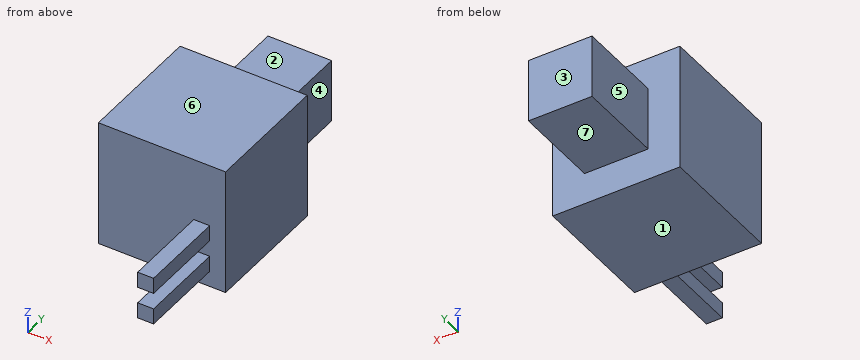
```python
from build123d import *

# Parameters (mm, degrees)
SKETCH1_W           = 8
SKETCH1_H           = 8
BOSS_EXTRUDE1_DEPTH = 8
SKETCH2_W           = 4
SKETCH2_H           = 4
BOSS_EXTRUDE2_DEPTH = 5.5
SKETCH3_W           = 1
SKETCH3_H           = 1
BOSS_EXTRUDE3_DEPTH = 5.5


with BuildPart() as part:
    # Sketch1 → Boss-Extrude1 (new body)
    with BuildSketch(Plane(origin=(0, 0, 0), x_dir=(1, 0, 0), z_dir=(0, 1, 0))):
        Rectangle(SKETCH1_W, SKETCH1_H)
    extrude(amount=BOSS_EXTRUDE1_DEPTH)

    # Sketch2 → Boss-Extrude2 (add)
    with BuildSketch(Plane(origin=(0, 8, 0), x_dir=(1, 0, 0), z_dir=(0, 1, 0))):
        Rectangle(SKETCH2_W, SKETCH2_H)
    extrude(amount=BOSS_EXTRUDE2_DEPTH)

    # Sketch3 → Boss-Extrude3 (add)
    with BuildSketch(Plane.XZ):
        with Locations((2.5, -2.5)):
            Rectangle(SKETCH3_W, SKETCH3_H)
        with Locations((2.5, -0.47334968)):
            Rectangle(SKETCH3_W, SKETCH3_H)
    extrude(amount=BOSS_EXTRUDE3_DEPTH)


solid = part.part
```
Could you check a few things on this model? Use its own coordinates, in mm. Face numbers are marked on the shaded views. A direction names the side the tool comes from. Coordinates: 2 decimals unless noted, no trailing zeros. Write each loop counter-clockwise with the first axis right and the second up, starting at its lowest first coordinate (ties: lowest second). Pieces come first, ordered by that corner, then holes. Notation, with made-up numbers: (40.5, 12) -> (92.5, 12) arc R32 ccw to (92.5, 46) -> close; hole circle Ø10 at (38.5, -14.75). An arc over 180 degrees is marked (long way). Write item = value, one per line. Start each with the question number.
(1) I want a section at B-B (z = -1.75). Please give me the cut outline in (x, y), plus the area to 3 significant figures.
(2) I want a section at A-A (x = 0). Please give me the cut outline in (y, z), plus the area to 3 significant figures.
(3) Which directions (+Z, -Z, +X, -X, +Y, -Y) give clear straight access to the entire face, cutting with the end or side of a thin tool? Please do the marked faces 4, 5, 6 and 7.
(4) I want a section at D-D (z = -0.25). Please give me the cut outline in (x, y), plus the area to 3 significant figures.
(5) I need wall thicknesses on line 1 (X direction, y = 10, z = 1); line 2 (Y direction, x = 2.5, z = -2.5); line 3 (Y direction, x = 0.75, z = 1). Which ranges of each line are inside material? Lowest first, please. Write a range as [from, to].
(6) I want a section at C-C (y = 11.75). Please give me the cut outline in (x, z), plus the area to 3 significant figures.
(7) We'd pull the mould along Z, two halves only. Please class the marked faces 1, 2 and 3: released by +Z, released by -Z, zero draft, split by the parting line, or undercut.
(8) Will these pins go through, and if not, where does the flat tip stop? pin 1 (2 mm diameter, centred on x = 0.5, y = 11.5, fed in from +Z); pin 2 (0.5 mm diameter, centred on x = 2.5, y = -1.5, fed in from -Z); pin 3 (0.8 mm diameter, centred on x = 2.5, y = -3, fed in from +Z).
Result set:
q1.outline = (-4, 0) -> (4, 0) -> (4, 8) -> (2, 8) -> (2, 13.5) -> (-2, 13.5) -> (-2, 8) -> (-4, 8) -> close
q1.area = 86.0 mm2
q2.outline = (0, -4) -> (8, -4) -> (8, -2) -> (13.5, -2) -> (13.5, 2) -> (8, 2) -> (8, 4) -> (0, 4) -> close
q2.area = 86.0 mm2
q3.face_4 = +Z, -Z, +X, +Y
q3.face_5 = +Z, -Z, -X, +Y
q3.face_6 = +Z, +X, -X, +Y, -Y
q3.face_7 = -Z, +X, -X, +Y
q4.outline = (-4, 0) -> (2, 0) -> (2, -5.5) -> (3, -5.5) -> (3, 0) -> (4, 0) -> (4, 8) -> (2, 8) -> (2, 13.5) -> (-2, 13.5) -> (-2, 8) -> (-4, 8) -> close
q4.area = 91.5 mm2
q5.line_1 = [-2, 2]
q5.line_2 = [-5.5, 8]
q5.line_3 = [0, 13.5]
q6.outline = (-2, -2) -> (2, -2) -> (2, 2) -> (-2, 2) -> close
q6.area = 16.0 mm2
q7.face_1 = released by -Z
q7.face_2 = released by +Z
q7.face_3 = zero draft
q8.pin_1 = 2
q8.pin_2 = -3
q8.pin_3 = 0.03
